Input: dimensioned drawing with shaded views. Units: mm. Origin: part minimum x, y, z. Coordinates: 2 decimals unless noted, no trailing zeros. Loops run counter-clockwise (first coordinate to the right, second up) from the corner with the lowest first, then second, coordinate; pieces in that order, holes last. Notation, with made-up numbers: (69, 1.5) -> (119, 1.5) arc R15 ccw to (119, 14.5) -> close; hole circle Ø7 at (-23, 41). An arc over 180 degrees is marked (long way). Answer as CSV lines item,"result".
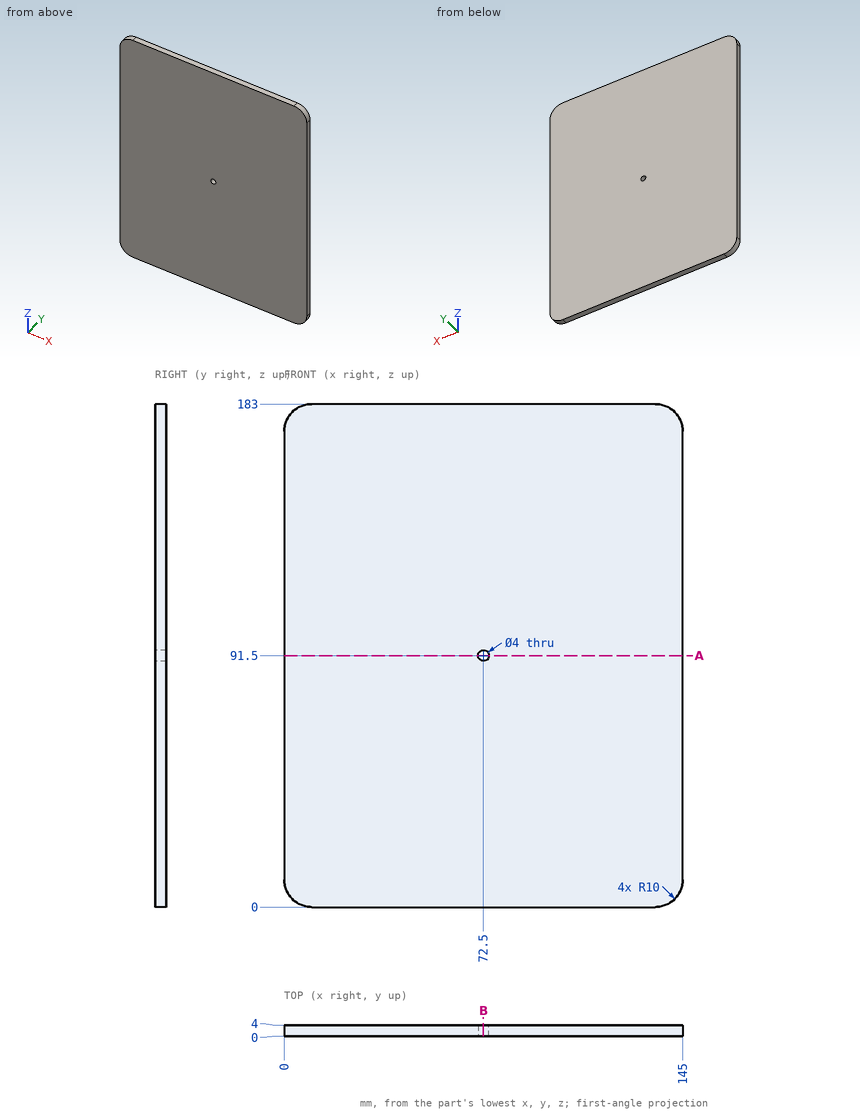
(1) Pin query (flat end, axial travel): pin 1 Ø6 at (x, z) = (66.5, 19.5) entering from -Y; pin 2 Ø2.5 at (x, z) = (72.5, 91.5) entering from +Y. Return the tip coordinate at first contact, or that it passes through.
Computed values:
pin 1,"y = 0"
pin 2,"through"
(2) Material intervals for L1, parallel to Z at x = 72.5, y = 1.3; L2, parallel to X at y = 1.7, z = 91.5; L3, parallel to Z at x = 138, y = 2.45, sorted ascending. Write a range as [from, to].
Computed values:
L1,"[0, 89.5], [93.5, 183]"
L2,"[0, 70.5], [74.5, 145]"
L3,"[0.46, 182.54]"
(3) Cut plane B-B (x = 72.5). Return the cut outline in (y, z), then the cut area to 3 significant figures.
Computed values:
outline,"(0, 0) -> (4, 0) -> (4, 89.5) -> (0, 89.5) -> close; (0, 93.5) -> (4, 93.5) -> (4, 183) -> (0, 183) -> close"
area,"716 mm^2"
(4) Cut plane A-A (z = 91.5). Return the cut outline in (x, y).
Computed values:
outline,"(0, 0) -> (70.5, 0) -> (70.5, 4) -> (0, 4) -> close; (74.5, 0) -> (145, 0) -> (145, 4) -> (74.5, 4) -> close"
